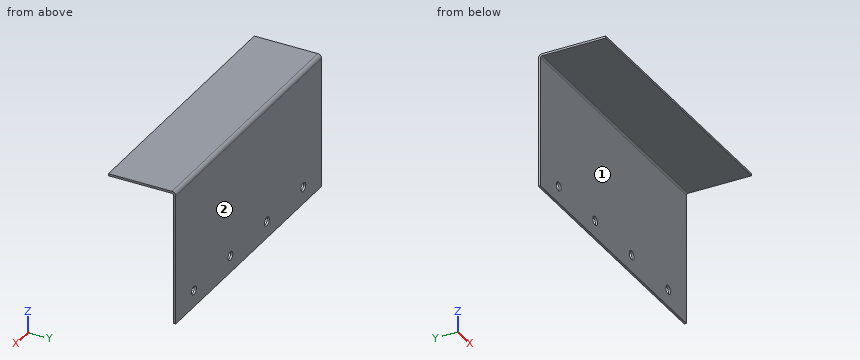
Autodesk Inventor part; units mm, degrees
ref_plane "YZ Plane" through (0, 0, 0) normal (1, 0, 0) x (0, 1, 0)
ref_plane "XZ Plane" through (0, 0, 0) normal (0, 1, 0) x (-1, 0, 0)
ref_plane "XY Plane" through (0, 0, 0) normal (0, 0, 1) x (1, 0, 0)
sketch "Sketch1" plane through (0, 0, 0) normal (0, 1, 0) x (-1, 0, 0)
  line L0 (0, 0) -> (203.2, 0)
  line L1 (203.2, 0) -> (203.2, 25.4)
  line L2 (203.2, 25.4) -> (0, 25.4) construction
  line L3 (0, 25.4) -> (0, 0)
  line L4 (25.4, 12.7) -> (76.2, 12.7) construction
  circle A0 centre (25.4, 12.7) radius 3.302
  circle A1 centre (76.2, 12.7) radius 3.302
  line L5 (50.8, 25.4) -> (50.8, 0) construction
  circle A2 centre (127, 12.7) radius 3.302
  circle A3 centre (177.8, 12.7) radius 3.302
  line L6 (127, 12.7) -> (177.8, 12.7) construction
  line L7 (152.4, 25.4) -> (152.4, 0) construction
  line L8 (0, 25.4) -> (0, 101.6)
  line L9 (0, 101.6) -> (203.2, 101.6)
  line L10 (203.2, 101.6) -> (203.2, 25.4)
  point P0 (50.8, 12.7)
  point P1 (152.4, 12.7)
  dimension "d0" = 50.8
  dimension "d1" = 6.604
  dimension "d2" = 6.604
  dimension "d3" = 25.4
  dimension "d4" = 50.8
  dimension "d6" = 50.8
  dimension "d7" = 50.8
  dimension "d8" = 76.2
  dimension "d9" = 203.2
extrude "Plate1" add sketch "Sketch1" along normal blind 1.5875
sketch "Sketch2" plane through (-203.2, 1.5875, 100.0125) normal (0, 0, 1) x (1, 0, 0)
  line L0 (203.2, 0) -> (0, 0)
  line L1 (0, 0) -> (0, -50.8)
  line L2 (0, -50.8) -> (203.2, -50.8)
  line L3 (203.2, -50.8) -> (203.2, 0)
edge flange "Flange1" height 50.8 angle 90 thickness 1.5875 bend radius 1.27 thickness toward (0, 0, 1) relief tear relief width 1.5875 relief depth 0.7937 edges at (-101.6, 0, 101.6) wall of the first edge with corners at (0, 1.5875, 100.0125) (-203.2, 1.5875, 100.0125) (-203.2, -49.2125, 100.0125) (0, -49.2125, 100.0125)
bend "Bend1"
corner "Corner1"
equation "\"d11\" = BendReliefWidth"
equation "\"d12\" = BendReliefDepth"
equation "\"d13\" = MinimumRemnant"
equation "\"d14\" = BendRadius"
equation "\"d18\" = CornerReliefSize"
equation "\"d19\" = GapSize"
equation "\"d20\" = JacobiRadiusSize"
equation "\"BendRadius\" = Thickness"
equation "\"BendReliefWidth\" = Thickness"
equation "\"BendReliefDepth\" = 0.5 * Thickness"
equation "\"CornerReliefSize\" = 4 * Thickness"
equation "\"MinimumRemnant\" = 2 * Thickness"
equation "\"TransitionRadius\" = BendRadius"
equation "\"JacobiRadiusSize\" = BendRadius"
equation "\"GapSize\" = Thickness"
equation "\"d10\" = BendRadius"
properties part number "Electrical Board Mount Part2" material "Aluminum 6061"
The listing builds one solid part. Answer for the finished solid, in the listing's coordinates (mm). Face numbers are marked on the shaded views. A direction names the side the tool comes from. Coordinates: 2 decimals unless noted, no trailing zeros. Loops run counter-clockwise (first coordinate to the right, second up) from the corner with the lowest first, then second, coordinate; pieces in that order, holes last.
1) Find the intervals of material crossed by L1, parallel to Y at x = -177.5, z = 43; L2, parallel to Z at x = -71, y = -36; L3, parallel to Z at x = -177.8, y = 0.55, in increasing order.
2) Find section D-D on z = 49. Write down the section's boundary in (x, y), then the cut area to 3 significant figures.
3) Find section A-A on x = -25.4. Write down the section's boundary in (y, z) (1 decimal).
4) A tool of negligible diameter and unlimited length cuts with its end or side. For the marked faces 1 and 2, from which of +Z, -Z, +X, -X, +Y, -Y can it reach the whole face along a straight path? Write none if from no direction.
5) Find section C-C on y = -26.5. Write down the section's boundary in (x, z).
6) Flat-ended cylindrical pins translate along their axes: pin 1 Ø3 at (x, z) = (-144.5, 52.5) entering from -Y; pin 2 Ø8.5 at (x, z) = (-76.2, 12.7) entering from +Y; pin 3 Ø5.5 at (x, z) = (-25.4, 12.7) entering from -Y; pin 4 Ø12 at (x, y) = (-126.5, -29) entering from -Z. Find the tip coordinate at first contact, or state that the pin passes through.
7) Find section B-B on x = -70. Write down the section's boundary in (y, z) (1 decimal).
Values:
1. L1: y = 0 to 1.59
1. L2: z = 100.01 to 101.6
1. L3: z = 0 to 9.4, 16 to 100.95
2. outline: (-203.2, 0) - (0, 0) - (0, 1.59) - (-203.2, 1.59) - close
2. area: 323 mm2
3. outline: (-49.2, 100) - (-1.3, 100) arc R1.3 cw to (0, 98.7) - (0, 16) - (1.6, 16) - (1.6, 98.7) arc R2.9 ccw to (-1.3, 101.6) - (-49.2, 101.6) - close; (0, 0) - (1.6, 0) - (1.6, 9.4) - (0, 9.4) - close
4. face 1: -Z, +X, -X, -Y
4. face 2: +Z, -Z, +X, -X, +Y
5. outline: (-203.2, 100.01) - (0, 100.01) - (0, 101.6) - (-203.2, 101.6) - close
6. pin 1: stops at y = 0
6. pin 2: stops at y = 1.59
6. pin 3: passes through
6. pin 4: stops at z = 100.01
7. outline: (-49.2, 100) - (-1.3, 100) arc R1.3 cw to (0, 98.7) - (0, 0) - (1.6, 0) - (1.6, 98.7) arc R2.9 ccw to (-1.3, 101.6) - (-49.2, 101.6) - close
